Check sheet for the modelled part. Datum: model origin and axes. Units: mm. Round coordinates to 2 decimals unless told otherwise and drop trailing zeros. Order: outer loops, then holes, each group sorted by start corner. A loop starts at its lowest first (then second) coordinate and runs counter-clockwise, first axis right, second up. Notation, with made-up numbers: (22.25, -29.5) -> (59.25, -29.5) arc R28 ccw to (59.25, 4.5) -> close; hole circle Ø7 at (4.25, 89.25). An arc over 180 degrees is marked (long way). Use CSV: the item, a comma, the result in double quotes.
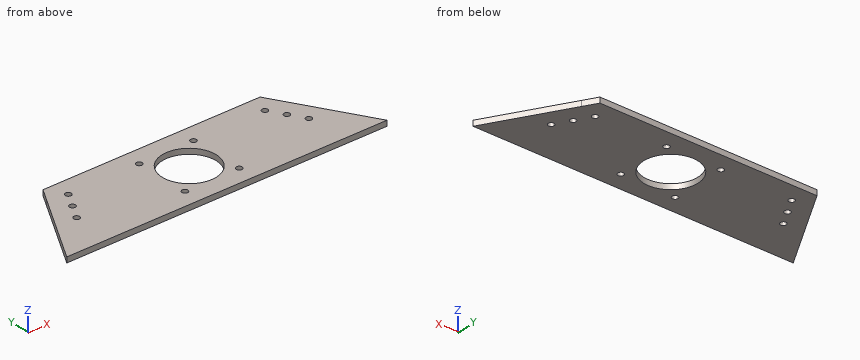
```python
from build123d import *

# Parameters (mm, degrees)
SKETCH_1_W          = 130
SKETCH_1_H          = 20
SKETCH_1_R          = 1.65
EXTRUDE_1_DEPTH     = 3
SKETCH_2_W          = 130
SKETCH_2_H          = 30
EXTRUDE_2_DEPTH     = 3
SKETCH_3_R          = 15
SKETCH_3_R_2        = 1.65
CUT_EXTRUDE_1_DEPTH = 3
CUT_EXTRUDE_2_DEPTH = 3
EXTRUDE_3_DEPTH     = 3
SKETCH_6_R          = 1.65
CUT_EXTRUDE_3_DEPTH = 3


with BuildPart() as part:
    # 草图1 → 凸台-拉伸1 (new body)
    with BuildSketch(Plane.XY):
        Rectangle(SKETCH_1_W, SKETCH_1_H)
        with Locations((-55, 0)):
            Circle(SKETCH_1_R, mode=Mode.SUBTRACT)
        with Locations((55, 0)):
            Circle(SKETCH_1_R, mode=Mode.SUBTRACT)
    extrude(amount=EXTRUDE_1_DEPTH)

    # 草图2 → 凸台-拉伸2 (add)
    with BuildSketch(Plane.XY.offset(3)):
        with Locations((0, -25)):
            Rectangle(SKETCH_2_W, SKETCH_2_H)
    extrude(amount=-EXTRUDE_2_DEPTH)

    # 草图3 → 切除-拉伸1 (cut)
    with BuildSketch(Plane.XY):
        with Locations((0, -15)):
            Circle(SKETCH_3_R)
        with Locations((-15.202795796, 0.202795796)):
            Circle(SKETCH_3_R_2)
        with Locations(Location((-15.202795796, -30.202795796, 0), (0, 0, 180))):
            Circle(SKETCH_3_R_2)
        with Locations((15.202795796, -30.202795796)):
            Circle(SKETCH_3_R_2)
        with Locations(Location((15.202795796, 0.202795796, 0), (0, 0, 180))):
            Circle(SKETCH_3_R_2)
    extrude(amount=CUT_EXTRUDE_1_DEPTH, mode=Mode.SUBTRACT)

    # 草图4 → 切除-拉伸2 (cut)
    with BuildSketch(Plane.XY):
        Polygon((65, 10), (60.77, 10), (65, 2.673425084), align=None)
        Polygon((-65, 2.673425084), (-65, 10), (-60.77, 10), align=None)
    extrude(amount=CUT_EXTRUDE_2_DEPTH, mode=Mode.SUBTRACT)

    # 草图5 → 凸台-拉伸3 (add)
    with BuildSketch(Plane.XY.offset(3)):
        Polygon((-65, 2.673425084), (-89.637513459, -40), (-65, -40), align=None)
        Polygon((89.637513459, -40), (65, -40), (65, 2.673425084), align=None)
    extrude(amount=-EXTRUDE_3_DEPTH)

    # 草图6 → 切除-拉伸3 (cut)
    with BuildSketch(Plane(origin=(0, 0, 0), x_dir=(-1, 0, 0), z_dir=(0, 0, -1))):
        with Locations((-60, -8.660254038)):
            Circle(SKETCH_6_R)
        with Locations((-65, -17.320508076)):
            Circle(SKETCH_6_R)
        with Locations(Location((65, -17.320508076, 0), (0, 0, 180))):
            Circle(SKETCH_6_R)
        with Locations(Location((60, -8.660254038, 0), (0, 0, 180))):
            Circle(SKETCH_6_R)
    extrude(amount=-CUT_EXTRUDE_3_DEPTH, mode=Mode.SUBTRACT)


solid = part.part
```
Q1. Sectioned sample at A-A, the plane x = 9. Enter the section's corners in (y, z), then the cut area to 3 significant figures.
Result sheet:
outline,"(-40, 0) -> (-27, 0) -> (-27, 3) -> (-40, 3) -> close; (-3, 0) -> (10, 0) -> (10, 3) -> (-3, 3) -> close"
area,"78.0 mm^2"
Q2. Sectioned sample at D-D, the plane x = 76. Enter the section's corners in (y, z), then the cut area to 3 significant figures.
Result sheet:
outline,"(-40, 0) -> (-16.38, 0) -> (-16.38, 3) -> (-40, 3) -> close"
area,"70.9 mm^2"
Q3. Scan lines: L1, parallel to Y at x = 55, z = 0.6; L2, parallel to Y at x = 65, z = 2.1; L3, parallel to X at y = -31, z = 0.95. Record each from-to range of solid material in increasing order.
Result sheet:
L1,"y = -40 to -1.65, 1.65 to 10"
L2,"y = -40 to -18.97, -15.67 to 2.67"
L3,"x = -84.44 to -16.65, -13.76 to 13.76, 16.65 to 84.44"
Q4. Sectioned sample at C-C, the plane z = 1.35. State how many separate pieces and enclosed holes the cut face has, then the cut area to 3 significant figures.
Result sheet:
separate pieces,"1"
enclosed holes,"11"
area,"6,730 mm^2"
Q5. Sectioned sample at B-B, the plane y = -22. Enter the section's corners in (x, z), then the cut area to 3 significant figures.
Result sheet:
outline,"(-79.25, 0) -> (-13.27, 0) -> (-13.27, 3) -> (-79.25, 3) -> close; (13.27, 0) -> (79.25, 0) -> (79.25, 3) -> (13.27, 3) -> close"
area,"396 mm^2"
Q6. Go/stop test with flat-tipped pins: pin 1 (4.5 mm diameter, centred on x = -65, y = -17.32, fed in from -Z); pin 2 (2.5 mm diameter, centred on x = 15.2, y = -30.2, fed in from +Z); pin 3 (1.5 mm diameter, centred on y = -4.5, z = 1, fed in from +X). Record where each tip stops, or that it passes through.
Result sheet:
pin 1,"stops at z = 0"
pin 2,"passes through"
pin 3,"stops at x = 69.57"
